Check sheet for the modelled part. Datum: model origin and axes. Units: mm. Give positions to 0.01 mm unless a question says otherwise; leave off trailing zeros. Loops run counter-clockwise (first coordinate to the right, second up) from the corner with the lowest first, then second, coordinate; pieces in that order, holes last. Notation, with made-up numbers: (-0.75, 15) - (51.25, 15) arc R27 ccw to (51.25, 34) - close; hole circle Ø7 at (-4.75, -17). An arc over 180 degrees is marked (long way). Use one line per item in the form item = value.
from build123d import *

# Parameters (mm, degrees)
BOSS_EXTRUDE1_DEPTH = 3.175
VARFILLET1_DEPTH    = 3.175
SKETCH2_R           = 17.4625
SKETCH2_R_2         = 7.9375
SKETCH2_R_3         = 9.525
SKETCH2_R_4         = 3.175
SKETCH2_R_5         = 3.2639
CUT_EXTRUDE1_DEPTH  = 3.175
SKETCH2_3_R         = 19.05
SKETCH2_3_R_2       = 17.4625
SKETCH2_3_R_3       = 11.1125
SKETCH2_3_R_4       = 7.9375
SKETCH2_3_R_5       = 12.7
SKETCH2_3_R_6       = 9.525
CUT_EXTRUDE2_DEPTH  = 0.9906
CIRPATTERN1_COUNT   = 3
CIRPATTERN2_COUNT   = 3


with BuildPart() as part:
    # Sketch1 → Boss-Extrude1 (new body)
    with BuildSketch(Plane(origin=(0, 0, 0), x_dir=(1, 0, 0), z_dir=(0, 1, 0))):
        with BuildLine():
            Line((-38.1, 146.05), (-38.1, 21.997045256))
            Line((-38.1, 21.997045256), (-145.533010223, -40.029432116))
            ThreePointArc((-145.533010223, -40.029432116), (-159.478578107, -92.075), (-107.433010223, -106.020567884))
            Line((-107.433010223, -106.020567884), (0, -43.994090512))
            Line((0, -43.994090512), (107.433010223, -106.020567884))
            ThreePointArc((107.433010223, -106.020567884), (159.478578107, -92.075), (145.533010223, -40.029432116))
            Line((145.533010223, -40.029432116), (38.1, 21.997045256))
            Line((38.1, 21.997045256), (38.1, 146.05))
            ThreePointArc((38.1, 146.05), (0, 184.15), (-38.1, 146.05))
        make_face()
    extrude(amount=BOSS_EXTRUDE1_DEPTH)

    # VarFillet1: read off the stored shape, not the designer's step
    # VarFillet1 outline → VarFillet1 (add)
    with BuildSketch(Plane(origin=(0, 0, 0), x_dir=(1, 0, 0), z_dir=(0, 1, 0))):
        with BuildLine():
            add(Edge.make_bspline(
                [(6.35, -47.660264722), (0, -43.994090512), (-6.35, -47.660264722)],
                knots=[0, 0, 0, 1, 1, 1], degree=2, weights=[1, 0.866025404, 1]))
            Line((6.35, -47.660264722), (0, -43.994090512))
            Line((0, -43.994090512), (-6.35, -47.660264722))
        make_face()
        with BuildLine():
            add(Edge.make_bspline(
                [(-44.45, 18.330871047), (-38.1, 21.997045256), (-38.1, 29.329393675)],
                knots=[0, 0, 0, 1, 1, 1], degree=2, weights=[1, 0.866025404, 1]))
            Line((-44.45, 18.330871047), (-38.1, 21.997045256))
            Line((-38.1, 21.997045256), (-38.1, 29.329393675))
        make_face()
        with BuildLine():
            add(Edge.make_bspline(
                [(38.1, 29.329393675), (38.1, 21.997045256), (44.45, 18.330871047)],
                knots=[0, 0, 0, 1, 1, 1], degree=2, weights=[1, 0.866025404, 1]))
            Line((38.1, 29.329393675), (38.1, 21.997045256))
            Line((38.1, 21.997045256), (44.45, 18.330871047))
        make_face()
    extrude(amount=VARFILLET1_DEPTH)

    # Sketch2 → Cut-Extrude1 (cut)
    with BuildSketch(Plane(origin=(0, 3.175, 0), x_dir=(1, 0, 0), z_dir=(0, 1, 0))):
        with Locations(Location((0, 0, 0), (0, 0, 270))):
            Circle(SKETCH2_R)
        with Locations(Location((0, 50.8, 0), (0, 0, 270))):
            Circle(SKETCH2_R_2)
        with Locations(Location((0, 101.6, 0), (0, 0, 270))):
            Circle(SKETCH2_R_2)
        with Locations(Location((0, 139.7, 0), (0, 0, 270))):
            Circle(SKETCH2_R_3)
        with Locations(Location((0, 179.705, 0), (0, 0, 270))):
            Circle(SKETCH2_R_4)
        with Locations(Location((0, 171.45, 0), (0, 0, 270))):
            Circle(SKETCH2_R_5)
        with Locations(Location((-25.4, 85.09, 0), (0, 0, 270))):
            Circle(SKETCH2_R_5)
        with Locations(Location((25.4, 85.09, 0), (0, 0, 270))):
            Circle(SKETCH2_R_5)
    cut_extrude1 = extrude(amount=-CUT_EXTRUDE1_DEPTH, mode=Mode.SUBTRACT)

    # Sketch2_3 → Cut-Extrude2 (cut)
    # profile 1 of 4: a face of its own
    with BuildSketch(Plane(origin=(0, 3.175, 0), x_dir=(1, 0, 0), z_dir=(0, 1, 0))):
        with Locations(Location((0, 0, 0), (0, 0, 270))):
            Circle(SKETCH2_3_R)
        with Locations(Location((0, 0, 0), (0, 0, 270))):
            Circle(SKETCH2_3_R_2, mode=Mode.SUBTRACT)
    # profile 2 of 4: a face of its own
    with BuildSketch(Plane(origin=(0, 3.175, 0), x_dir=(1, 0, 0), z_dir=(0, 1, 0))):
        with Locations(Location((0, 50.8, 0), (0, 0, 270))):
            Circle(SKETCH2_3_R_3)
        with Locations(Location((0, 50.8, 0), (0, 0, 270))):
            Circle(SKETCH2_3_R_4, mode=Mode.SUBTRACT)
    # profile 3 of 4: a face of its own
    with BuildSketch(Plane(origin=(0, 3.175, 0), x_dir=(1, 0, 0), z_dir=(0, 1, 0))):
        with Locations(Location((0, 101.6, 0), (0, 0, 270))):
            Circle(SKETCH2_3_R_3)
        with Locations(Location((0, 101.6, 0), (0, 0, 270))):
            Circle(SKETCH2_3_R_4, mode=Mode.SUBTRACT)
    # profile 4 of 4: a face of its own
    with BuildSketch(Plane(origin=(0, 3.175, 0), x_dir=(1, 0, 0), z_dir=(0, 1, 0))):
        with Locations(Location((0, 139.7, 0), (0, 0, 270))):
            Circle(SKETCH2_3_R_5)
        with Locations(Location((0, 139.7, 0), (0, 0, 270))):
            Circle(SKETCH2_3_R_6, mode=Mode.SUBTRACT)
    cut_extrude2 = extrude(amount=-CUT_EXTRUDE2_DEPTH, mode=Mode.SUBTRACT)

    # CirPattern1: Cut-Extrude1 ×3 about axis
    cirpattern1_axis = Axis((0, 0, 0), (0, 1, 0))
    for i in range(1, CIRPATTERN1_COUNT):
        add(cut_extrude1.rotate(cirpattern1_axis, i * 360 / CIRPATTERN1_COUNT), mode=Mode.SUBTRACT)

    # CirPattern2: Cut-Extrude2 ×3 about axis
    cirpattern2_axis = Axis((0, 0, 0), (0, 1, 0))
    for i in range(1, CIRPATTERN2_COUNT):
        add(cut_extrude2.rotate(cirpattern2_axis, i * 360 / CIRPATTERN2_COUNT), mode=Mode.SUBTRACT)


solid = part.part
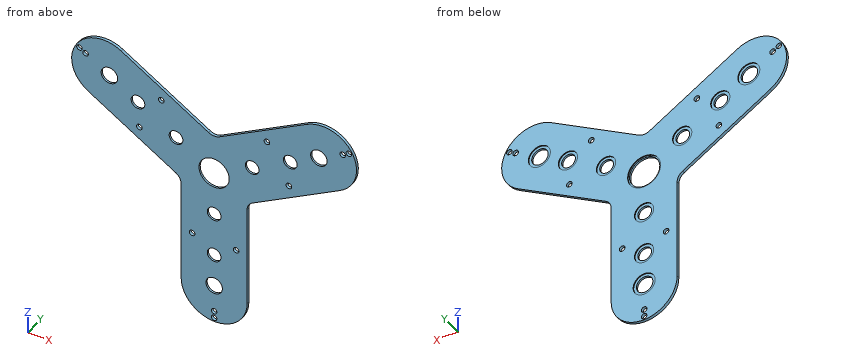
Item 1: Gauge pin test, flat ends, axial feed: P1, Ø2, axis at x = -82, z = 54.5, coming from the -Y side; P2, Ø12.5, axis at x = 117, z = 70.5, coming from the +Y side. Record the tip position at first contact, or that the pin passes through.
Answer block:
P1 = 0
P2 = 2.18
Item 2: Section check C-C on y = 1.1. Give the number of separate pieces and of enclosed holes in the cut face, then the cut area to 3 significant figures.
Answer block:
separate_pieces = 1
enclosed_holes = 22
area = 34,300 mm2
Item 3: Section check A-A on z = -101.6. Record the boundary of the cut face in (x, y) (1 decimal), then the cut area to 3 significant figures.
Answer block:
outline = (-38.1, 0) - (-7.9, 0) - (-7.9, 2.2) - (-11.1, 2.2) - (-11.1, 3.2) - (-38.1, 3.2) - close; (7.9, 0) - (38.1, 0) - (38.1, 3.2) - (11.1, 3.2) - (11.1, 2.2) - (7.9, 2.2) - close
area = 185 mm2
Item 4: Thickness scan on L1, parallel to X at y = 2.85, z = 69.85; L2, parallel to X at y = 1.8, z = 44; L3, parallel to X at y = 3, z = -33. Record the ranges inside material, lowest first.
Answer block:
L1 = -164.45 to -133.68, -108.28 to -44.78, 44.78 to 108.28, 133.68 to 164.45
L2 = -151.16 to -92.08, -83.89 to 83.89, 92.08 to 151.16
L3 = -38.1 to 38.1
Item 5: Section check B-B on z = -139.7. Record the boundary of the cut face in (x, y) (3 decimals), then the cut area to 3 significant figures.
Answer block:
outline = (-38.1, 0) - (-9.525, 0) - (-9.525, 2.184) - (-12.7, 2.184) - (-12.7, 3.175) - (-38.1, 3.175) - close; (9.525, 0) - (38.1, 0) - (38.1, 3.175) - (12.7, 3.175) - (12.7, 2.184) - (9.525, 2.184) - close
area = 175 mm2
